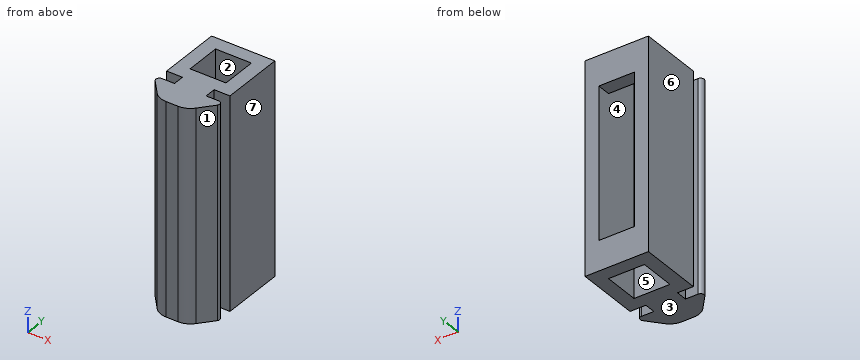
```python
from build123d import *

# Parameters (mm, degrees)
SKETCH1_W           = 10.2
SKETCH1_H           = 10.2
BOSS_EXTRUDE3_DEPTH = 60
FILLET1_R           = 1
FILLET2_R           = 5
SKETCH2_W           = 10.2
SKETCH2_H           = 43
CUT_EXTRUDE1_DEPTH  = 10


with BuildPart() as part:
    # Sketch1 → Boss-Extrude3 (new body)
    # profile 1 of 2: a face of its own
    with BuildSketch(Plane.XY):
        Polygon((-9, 10.5), (-4.5, 10.5), (4.5, 10.5), (9, 10.5), (9, 28.5), (-9, 28.5), align=None)
        with Locations((0, 19.5)):
            Rectangle(SKETCH1_W, SKETCH1_H, mode=Mode.SUBTRACT)
    # profile 2 of 2: a face of its own
    with BuildSketch(Plane.XY):
        Polygon((-4.5, 7.3), (-10.25, 7.3), (-4, 0), (4, 0), (10.25, 7.3), (4.5, 7.3), (4.5, 10.5), (-4.5, 10.5), align=None)
    extrude(amount=BOSS_EXTRUDE3_DEPTH)

    # Fillet1
    fillet1_edges = [part.edges().sort_by_distance(p)[0] for p in [
        (10.25, 7.3, 30),
        (-10.25, 7.3, 30),
    ]]
    fillet(fillet1_edges, radius=FILLET1_R)

    # Fillet2
    fillet2_edges = [part.edges().sort_by_distance(p)[0] for p in [
        (4, 0, 30),
        (-4, 0, 30),
    ]]
    fillet(fillet2_edges, radius=FILLET2_R)

    # Sketch2 → Cut-Extrude1 (cut)
    with BuildSketch(Plane(origin=(0, 28.5, 0), x_dir=(1, 0, 0), z_dir=(0, 1, 0))):
        with Locations((0, -30)):
            Rectangle(SKETCH2_W, SKETCH2_H)
    extrude(amount=-CUT_EXTRUDE1_DEPTH, mode=Mode.SUBTRACT)


solid = part.part
```
Design review of the part built by this model. Coordinates are the model's own, in mm. Face numbers are marked on the shaded views. A direction names the side the tool comes from. Give positions to 0.01 mm unless a question says otherwise; leave off trailing zeros. Order: outer loops, then holes, each group sorted by start corner. A loop starts at its lowest first (then second) coordinate and runs counter-clockwise, first axis right, second up. Notation, with made-up numbers: (7.5, 26.25) -> (44.5, 26.25) arc R34 ccw to (44.5, 57.25) -> close; hole circle Ø6 at (-2, -14). An arc over 180 degrees is marked (long way). Write item = value, one per line. Start each with the question number.
(1) We need section C-C on y = 21.25. Write out the cut boundary in (x, z).
(2) We need section B-B on z = 52.5. Write out the cut boundary in (x, y), plus the area to 3 significant figures.
(3) To check wall thickness, follow line 1 along X through (y, z) = (17, 10); line 2 along Y through (x, z) = (-5, 4.5); line 3 along Y through (x, z) = (0, 4). State the ranges of each line that lie inside material, in increasing order.
(4) For the marked faces 4, 5, 6 and 7, list the 3-axis set-ups (+Z, -Z, +X, -X, +Y, -Y) from which the entire face can be reached by the end or side of a thin tool; tool diameter is ignored.
(5) For pin 1 (8 mm diameter, centred on x = -1.5, z = 29, fed in from +Y); pin 2 (6 mm diameter, centred on x = -7, z = 39.5, fed in from -Y); pin 3 (1.5 mm diameter, centred on y = 12.5, z = 30.5, fed in from -X); pin 4 (14.5 mm diameter, centred on y = 16, z = 24.5, fed in from +X), all flat-tipped, find the tip position at first contact; note any pin that passes through.
(6) Mouldability with a two-part tool opening along X and no side actions: class the marked faces 1, 2 and 3 as +X half, -X half, draft (parallel to the pull), parting line (faces both ways), or undercut.
(7) We need section D-D on x = 6.5. Write out the cut boundary in (y, z).
(8) We need section A-A on x = 0. Write out the cut boundary in (y, z), plus the area to 3 significant figures.
Numbers:
q1.outline = (-9, 0) -> (-5.1, 0) -> (-5.1, 60) -> (-9, 60) -> close; (5.1, 0) -> (9, 0) -> (9, 60) -> (5.1, 60) -> close
q2.outline = (-9, 10.5) -> (-4.5, 10.5) -> (-4.5, 7.3) -> (-8.08, 7.3) arc R1 ccw to (-8.84, 5.65) -> (-5.5, 1.75) arc R5 ccw to (-1.7, 0) -> (1.7, 0) arc R5 ccw to (5.5, 1.75) -> (8.84, 5.65) arc R1 ccw to (8.08, 7.3) -> (4.5, 7.3) -> (4.5, 10.5) -> (9, 10.5) -> (9, 28.5) -> (-9, 28.5) -> close; hole (-5.1, 14.4) -> (5.1, 14.4) -> (5.1, 24.6) -> (-5.1, 24.6) -> close
q2.area = 349 mm^2
q3.line_1 = -9 to -5.1, 5.1 to 9
q3.line_2 = 1.24 to 7.3, 10.5 to 14.4, 24.6 to 28.5
q3.line_3 = 0 to 14.4, 24.6 to 28.5
q4.face_4 = none
q4.face_5 = +Z, -Z
q4.face_6 = +Z, -Z, -X, +Y
q4.face_7 = +Z, -Z, +X, +Y
q5.pin_1 = 28.5
q5.pin_2 = 0.56
q5.pin_3 = -9
q5.pin_4 = 9
q6.face_1 = +X half
q6.face_2 = undercut
q6.face_3 = draft
q7.outline = (2.92, 0) -> (7.3, 0) -> (7.3, 60) -> (2.92, 60) -> close; (10.5, 0) -> (28.5, 0) -> (28.5, 60) -> (10.5, 60) -> close
q8.outline = (0, 0) -> (14.4, 0) -> (14.4, 60) -> (0, 60) -> close; (24.6, 0) -> (28.5, 0) -> (28.5, 8.5) -> (24.6, 8.5) -> close; (24.6, 51.5) -> (28.5, 51.5) -> (28.5, 60) -> (24.6, 60) -> close
q8.area = 930 mm^2
